Geometry check sheet. Reference: drawing and pictorial views, mm from the part's lowest x, y, z. Give positions to 0.01 mm unless a question says otherwise; leave off trailing zeros. Order: outer loops, then holes, each group sorted by start corner. A loop starts at its lowest first (then second) coordinate and runs counter-clockwise, first axis right, second up. Notation, with made-up numbers: (-3.5, -21) - (35.5, -21) arc R19 cw to (35.5, 5) - close; hole circle Ø3 at (11, 47). An arc over 180 degrees is marked (long way). Answer in a Markdown table with one row per item.
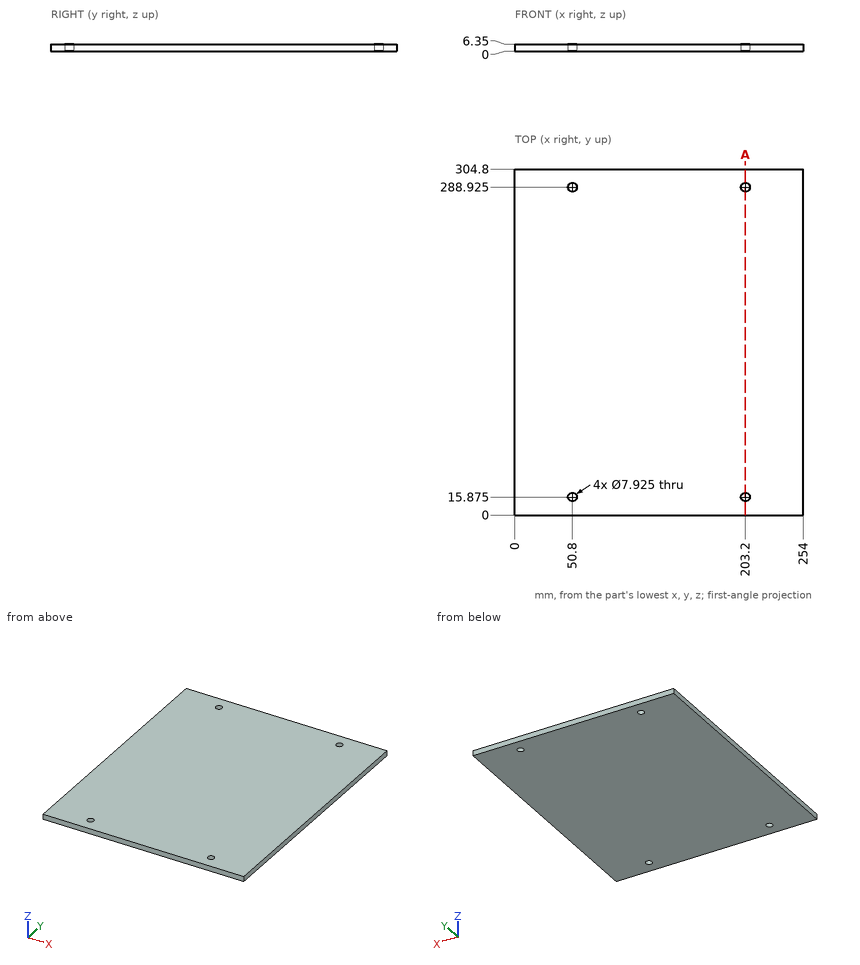
(1) Thickness scan on L1, parallel to Y at x = 203.2, z = 2; L2, parallel to X at y = 18.5, z = 5. Record the ranges inside material, lowest first.
Geometry says:
| item | result |
|---|---|
| L1 | 0 to 11.91, 19.84 to 284.96, 292.89 to 304.8 |
| L2 | 0 to 47.83, 53.77 to 200.23, 206.17 to 254 |
(2) Cross-section at A-A, the plane x = 203.2. Record the cut outline in (y, z), then the cut area to 4 significant figures.
Geometry says:
| item | result |
|---|---|
| outline | (0, 0) - (11.91, 0) - (11.91, 6.35) - (0, 6.35) - close; (19.84, 0) - (284.96, 0) - (284.96, 6.35) - (19.84, 6.35) - close; (292.89, 0) - (304.8, 0) - (304.8, 6.35) - (292.89, 6.35) - close |
| area | 1,835 mm² |
(3) Gauge pin test, flat end, axial feed: P1, Ø7, axis at x = 50.8, y = 15.875, coming from the -Z side. Record the tip position at first contact, or that the pin passes through.
Geometry says:
| item | result |
|---|---|
| P1 | through |
